```python
from build123d import *

# Parameters (mm, degrees)
SKETCH1_R           = 10.875
SKETCH1_R_2         = 1.625
BOSS_EXTRUDE1_DEPTH = 5
SKETCH1_2_R         = 10.875
BOSS_EXTRUDE2_DEPTH = 17
CHAMFER1_SIZE       = 0.8
SKETCH3_R           = 2.875
CUT_EXTRUDE1_DEPTH  = 3
CHAMFER2_SIZE       = 0.4


with BuildPart() as part:
    # Sketch1 → Boss-Extrude1 (new body)
    with BuildSketch(Plane(origin=(0, 0, 0), x_dir=(1, 0, 0), z_dir=(0, 1, 0))):
        with BuildLine():
            ThreePointArc((5.599866179, 18.468846749), (0, 24.625), (-5.599866179, 18.468846749))
            ThreePointArc((-5.599866179, 18.468846749), (-6.125206634, 15.721438867), (-8.043986082, 13.686121179))
            ThreePointArc((-8.043986082, 13.686121179), (-13.748153285, 7.9375), (-15.874521661, 0.123235705))
            ThreePointArc((-15.874521661, 0.123235705), (-16.67776876, -2.556134885), (-18.794423553, -4.384797006))
            ThreePointArc((-18.794423553, -4.384797006), (-21.325875568, -12.3125), (-13.194557374, -14.084049744))
            ThreePointArc((-13.194557374, -14.084049744), (-10.552562126, -13.165303982), (-7.830535579, -13.809356884))
            ThreePointArc((-7.830535579, -13.809356884), (0, -15.875), (7.830535579, -13.809356884))
            ThreePointArc((7.830535579, -13.809356884), (10.552562126, -13.165303982), (13.194557374, -14.084049744))
            ThreePointArc((13.194557374, -14.084049744), (21.325875568, -12.3125), (18.794423553, -4.384797006))
            ThreePointArc((18.794423553, -4.384797006), (16.67776876, -2.556134885), (15.874521661, 0.123235705))
            ThreePointArc((15.874521661, 0.123235705), (13.748153285, 7.9375), (8.043986082, 13.686121179))
            ThreePointArc((8.043986082, 13.686121179), (6.125206634, 15.721438867), (5.599866179, 18.468846749))
        make_face()
        Circle(SKETCH1_R, mode=Mode.SUBTRACT)
        with Locations((0, 19)):
            Circle(SKETCH1_R_2, mode=Mode.SUBTRACT)
        with Locations((16.454482672, -9.5)):
            Circle(SKETCH1_R_2, mode=Mode.SUBTRACT)
        with Locations((-16.454482672, -9.5)):
            Circle(SKETCH1_R_2, mode=Mode.SUBTRACT)
    extrude(amount=BOSS_EXTRUDE1_DEPTH)

    # Sketch1<2> → Boss-Extrude2 (add)
    with BuildSketch(Plane(origin=(0, 0, 0), x_dir=(1, 0, 0), z_dir=(0, 1, 0))):
        Circle(SKETCH1_2_R)
    extrude(amount=BOSS_EXTRUDE2_DEPTH)

    # Sketch2 → Revolve1 (revolve)
    with BuildSketch(Plane.XY):
        Polygon((0, 17), (10.875, 17), (0, 32), align=None)
    revolve(axis=Axis((0, 18.413549721, 0), (0, -1, 0)))

    # Chamfer1
    chamfer1_edges = [part.edges().sort_by_distance(p)[0] for p in [
        (16.67776876, 0, 2.556134885),
        (21.325875568, 0, 12.3125),
        (10.552562126, 0, 13.165303982),
        (0, 0, 15.875),
        (-10.552562126, 0, 13.165303982),
        (-21.325875568, 0, 12.3125),
        (-16.67776876, 0, 2.556134885),
        (-13.748153285, 0, -7.9375),
        (-6.125206634, 0, -15.721438867),
        (0, 0, -24.625),
        (6.125206634, 0, -15.721438867),
        (13.748153285, 0, -7.9375),
    ]]
    chamfer(chamfer1_edges, length=CHAMFER1_SIZE)

    # Sketch3 → Cut-Extrude1 (cut)
    with BuildSketch(Plane.XZ):
        with Locations((0, -19)):
            Circle(SKETCH3_R)
        with Locations((-16.454482672, 9.5)):
            Circle(SKETCH3_R)
        with Locations((16.454482672, 9.5)):
            Circle(SKETCH3_R)
    extrude(amount=-CUT_EXTRUDE1_DEPTH, mode=Mode.SUBTRACT)

    # Chamfer2
    chamfer2_edges = [part.edges().sort_by_distance(p)[0] for p in [
        (-2.875, 0, -19),
        (-19.329482672, 0, 9.5),
        (13.579482672, 0, 9.5),
    ]]
    chamfer(chamfer2_edges, length=CHAMFER2_SIZE)


solid = part.part
```
Input: part model. Units: mm. Frame: model coordinates. A direction names the side the tool comes from. Round coordinates to 2 decimals unless told otherwise and drop trailing zeros. Loops run counter-clockwise (first coordinate to the right, second up) from the corner with the lowest first, then second, coordinate; pieces in that order, holes last. Notation, with made-up numbers: (17.25, 31) -> (56.25, 31) arc R14 ccw to (56.25, 44) -> close; hole circle Ø2 at (25, 30.5). An arc over 180 degrees is marked (long way). Use one line per item in the form item = value. Start each with the question number.
Item 1: Section query A-A on z = 9.5. Count the separate pieces of the cut face and the enclosed holes in it, then the cut area to 3 significant figures.
Item 2: Contact query for flat-ended pins moving along their axis: pin 1 Ø1.9 at (x, z) = (-16.45, 9.5) entering from -Y; pin 2 Ø1.7 at (x, z) = (0.5, -18) entering from -Y; pin 3 Ø1 at (x, z) = (-1, -4) entering from +Y; pin 4 Ø1.5 at (x, z) = (2.5, -18) entering from +Y. Output: stop coordinate, or through.
Item 3: Set-up query: faces 5 (the face through (-15, 3, 8)), 6 (the face through (-1.42, 10.92, -10.78)), 7 (the face through (-17, 3, 3)). Return all of +Z, -Z, +X, -X, +Y, -Y with unobstructed straight access to the full face (end or side cutting, diameter ignored); none if empty.
Item 4: Section query B-B on y = 15.5. Return the cut outline in (x, z) (3 decimals).
Item 5: Material intervals for L1, parallel to X at y = 4.3, z = -19 (3 decimals); L2, parallel to Y at x = -3, z = -13; L3, parallel to Z at x = 8.5, y = 10.5, sorted ascending. Write a range as from..to.
Item 6: Mould query, pull axis Z, two halves, no side actions, for faces 1 (the face through (-0.352, 3.986, -17.414)), 2 (the face through (0, 0, 0)), 3 (the face through (2.81, 27.94, 0.88)), 4 (the face through (0, 3, -21)). Classes: pulls with the +Z half, pulls with the -Z half, needs draft (parallel to the pull), parting line crosses it, or undercut.
Ans:
q1.separate_pieces = 3
q1.enclosed_holes = 0
q1.area = 313 mm^2
q2.pin_1 = through
q2.pin_2 = 3
q2.pin_3 = 27
q2.pin_4 = 5
q3.face_5 = -Y
q3.face_6 = +Y
q3.face_7 = -Z, -X, +Y, -Y
q4.outline = circle Ø21.75 at (0, 0)
q5.L1 = -5.625..-1.625, 1.625..5.625
q5.L2 = 0..5
q5.L3 = -6.78..6.78
q6.face_1 = undercut
q6.face_2 = needs draft
q6.face_3 = parting line crosses it
q6.face_4 = undercut
